Source: CAD feature listing. Evaluate the final solid. Frame: model axes, mm. Face numbers are marked on the shaded views. A direction names the side the tool comes from. Give positions to 0.01 mm unless a question says otherwise; leave off trailing zeros. Order: outer loops, then holes, each group sorted by start corner. A loop starts at its lowest first (then second) coordinate and runs counter-clockwise, first axis right, second up.
1) Section D-D, the plane y = 20. Return loops of the section in (x, z).
2) Section A-A, the plane z = 0. Give the number of separate pieces and of enclosed holes in the cut face, plus the area to 3 significant figures.
3) Section C-C, the plane z = -3.5. Return loops of the section in (x, y) (1 decimal), plus the area to 3 significant figures.
4) Access query for the marked faces 4, 5, 6, 7 and 8. Directions: +Z, -Z, +X, -X, +Y, -Y. A direction counts if a zero-diameter tool reaches every point of the face in a straight line with its end or side. Return the directions, or none.
5) Material intervals for line 1 (X direction, y = 19.95, z = 0); line 2 (Y direction, x = 12, z = -4.5); line 3 (Y direction, x = -7, z = 1) (3 decimals), sorted ascending.
6) Section B-B, the plane x = 14.5. Return loops of the section in (y, z), plus the area to 3 significant figures.
7) Draft query along Y for the marked faces 1, 2 and 3. Return one class per face: released by +Y, released by -Y, zero draft, split by the parting line, or undercut.
8) First-contact query: P1, Ø5, axis at x = 15, z = -0.5, coming from the -Y side; P2, Ø2, axis at y = 25, z = 2.5, coming from the +X side; P3, Ø4, axis at x = 15, z = 0.5, coming from the +Y side. Flat tips, straight axial feed; report the tip coordinate or a pass-through.
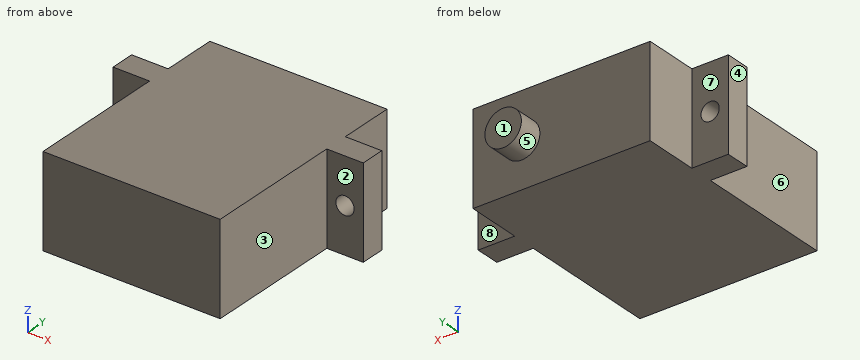
```python
from build123d import *

# Parameters (mm, degrees)
SKETCH2_W           = 23.114
SKETCH2_H           = 11.938
BOSS_EXTRUDE1_DEPTH = 28.575
SKETCH3_W           = 4.7625
SKETCH3_H           = 3.175
BOSS_EXTRUDE2_DEPTH = 11.938
SKETCH5_R           = 2.38125
BOSS_EXTRUDE3_DEPTH = 3.175
SKETCH8_R           = 1.190625
CUT_EXTRUDE1_DEPTH  = 28.590823072


with BuildPart() as part:
    # Sketch2 → Boss-Extrude1 (new body)
    with BuildSketch(Plane(origin=(0, 0, 0), x_dir=(1, 0, 0), z_dir=(0, 1, 0))):
        Rectangle(SKETCH2_W, SKETCH2_H)
    extrude(amount=BOSS_EXTRUDE1_DEPTH)

    # Sketch3 → Boss-Extrude2 (add, through all)
    with BuildSketch(Plane.XY.offset(5.969)):
        with Locations((13.93825, 19.84375)):
            Rectangle(SKETCH3_W, SKETCH3_H)
    boss_extrude2 = extrude(amount=-BOSS_EXTRUDE2_DEPTH)

    # Mirror1: Boss-Extrude2 across plane
    add(boss_extrude2.mirror(Plane(origin=(0, 0, 0), x_dir=(0, 0, 1), z_dir=(1, 0, 0))))

    # Sketch5 → Boss-Extrude3 (add)
    with BuildSketch(Plane(origin=(0, 28.575, 0), x_dir=(1, 0, 0), z_dir=(0, 1, 0))):
        with Locations(Location((5.207, 0, 0), (0, 0, 90))):
            Circle(SKETCH5_R)
    extrude(amount=BOSS_EXTRUDE3_DEPTH)

    # Sketch8 → Cut-Extrude1 (cut, through all)
    with BuildSketch(Plane(origin=(0, 21.43125, 0), x_dir=(1, 0, 0), z_dir=(0, 1, 0))):
        with Locations(Location((13.93825, 0, 0), (0, 0, 270))):
            Circle(SKETCH8_R)
    cut_extrude1 = extrude(amount=-CUT_EXTRUDE1_DEPTH, mode=Mode.SUBTRACT)

    # Mirror2: Cut-Extrude1 across plane
    add(cut_extrude1.mirror(Plane(origin=(0, 0, 0), x_dir=(0, 0, 1), z_dir=(1, 0, 0))), mode=Mode.SUBTRACT)


solid = part.part
```
From the geometry:
1. outline: (-16.32, -5.97) - (16.32, -5.97) - (16.32, 5.97) - (-16.32, 5.97) - close; hole circle Ø2.38 at (-13.94, 0); hole circle Ø2.38 at (13.94, 0)
2. separate pieces: 3
2. enclosed holes: 0
2. area: 691 mm2
3. outline: (-16.3, 18.3) - (-11.6, 18.3) - (-11.6, 0) - (11.6, 0) - (11.6, 18.3) - (16.3, 18.3) - (16.3, 21.4) - (11.6, 21.4) - (11.6, 28.6) - (-11.6, 28.6) - (-11.6, 21.4) - (-16.3, 21.4) - close
3. area: 691 mm2
4. face 4: +Z, -Z, -X, +Y, -Y
4. face 5: +Y
4. face 6: +Z, -Z, -X, -Y
4. face 7: +Z, -Z, -X, +Y
4. face 8: +Z, -Z, +X, +Y
5. line 1: x = -16.32 to -15.13, -12.75 to 12.75, 15.13 to 16.32
5. line 2: y = 18.26 to 21.43
5. line 3: y = 0 to 28.575
6. outline: (18.26, -5.97) - (21.43, -5.97) - (21.43, -1.05) - (18.26, -1.05) - close; (18.26, 1.05) - (21.43, 1.05) - (21.43, 5.97) - (18.26, 5.97) - close
6. area: 31.2 mm2
7. face 1: released by +Y
7. face 2: released by -Y
7. face 3: zero draft
8. P1: stops at y = 18.26
8. P2: stops at x = 11.56
8. P3: stops at y = 21.43
